The model under review builds one solid part; all positions refer to its coordinate system, in mm. A direction names the side the tool comes from. Coordinates: 2 decimals unless noted, no trailing zeros. Write each loop counter-clockwise with the first axis right and the second up, starting at its lowest first coordinate (ties: lowest second). Pieces come first, ordered by that corner, then holes.
1) Add section D-D, the plane y = 3.5. State the section outline as (x, z) points.
2) Machinability: for faces 5 (the flat face through (53, 4, 4.25)), 6 (the flat face through (53, 14.662, 3)), 7 (the flat face through (-9.287, 4, 1)), which of the approach directions +Z, -Z, +X, -X, +Y, -Y give a long, thin tool a straight path to every point of the face, cutting with its end or side? Answer none if there is none.
3) Mouldability with a two-part tool opening along Y and no side actions: class faces 1 (the flat face through (-3, 24.162, 6)), 2 (the cylindrical face through (-5.966, 30.025, 0.863)), 3 (the flat face through (24, 5, 0)), 4 (the cylindrical face through (52.034, 30.025, 0.863)) as released by +Y, released by -Y, zero draft, split by the parting line, or undercut.
4) For P1, Ø3, axis at x = 53.5, z = 3.5, coming from the -Y side; P2, Ø1, axis at x = 14.5, y = 16.5, coming from the -Z side; P3, Ø2.5, axis at x = -5.5, z = 7, coming from the -Y side; P4, Ø2, axis at x = 8.5, y = -7, coming from the +Z side, all flat-tipped, find the tip position at first contact; note any pin that passes through.
5) For line 1 (Z direction, x = 4, y = 11); line 2 (X direction, y = 15, z = 4.75); line 3 (X direction, y = -5, z = 1.5), list the stretches that pass through material, from the lowest coordinate up.
6) Add section A-A, the plane y = 20.5. State the section outline as (x, z) points.
7) Add section C-C, the plane x = 7. State the section outline as (y, z) points, then the cut area to 3 significant figures.
8) Add section B-B, the plane z = 2.5. State the section outline as (x, y) points.
from build123d import *

# Parameters (mm, degrees)
SKETCH003_W  = 5.5
SKETCH003_H  = 20.7
PAD002_DEPTH = 2.5
SKETCH_W     = 14
SKETCH_H     = 13.5
PAD001_DEPTH = 9
SKETCH002_R  = 1.375
PAD_DEPTH    = 1.75


with BuildPart() as displayport:
    # Sketch003 (on Face1 of ShapeBinder001) → Pad002 (new body)
    with BuildSketch(Plane.XY.offset(1.75)):
        with Locations((52.9627, 4.312003)):
            Rectangle(SKETCH003_W, SKETCH003_H)
    extrude(amount=PAD002_DEPTH)


with BuildPart() as usb:
    # Sketch (on Face1 of ShapeBinder) → Pad001 (new body)
    with BuildSketch(Plane.XY.offset(1.75)):
        with Locations((-3.2873, 17.412003)):
            Rectangle(SKETCH_W, SKETCH_H)
    extrude(amount=PAD001_DEPTH)


with BuildPart() as fusion001:
    # Sketch002 → Pad (new body)
    with BuildSketch(Plane.XY):
        with BuildLine():
            Line((-6.2873, 32.162003), (52.7127, 32.162003))
            ThreePointArc((55.7127, 29.162003), (54.83402, 31.283323), (52.7127, 32.162003))
            Line((55.7127, 29.162003), (55.7127, -20.837997))
            ThreePointArc((52.7127, -23.837997), (54.83402, -22.959317), (55.7127, -20.837997))
            Line((52.7127, -23.837997), (-6.2873, -23.837997))
            ThreePointArc((-9.2873, -20.837997), (-8.40862, -22.959317), (-6.2873, -23.837997))
            Line((-9.2873, -20.837997), (-9.2873, 29.162003))
            ThreePointArc((-6.2873, 32.162003), (-8.40862, 31.283323), (-9.2873, 29.162003))
        make_face()
        with Locations((-5.7873, 28.662003)):
            Circle(SKETCH002_R, mode=Mode.SUBTRACT)
        with Locations((-5.7873, -20.337997)):
            Circle(SKETCH002_R, mode=Mode.SUBTRACT)
        with Locations((52.2127, -20.337997)):
            Circle(SKETCH002_R, mode=Mode.SUBTRACT)
        with Locations((52.2127, 28.662003)):
            Circle(SKETCH002_R, mode=Mode.SUBTRACT)
    extrude(amount=PAD_DEPTH)

    # Fusion: union usb
    add(usb.part)

    # Fusion001: union displayport
    add(displayport.part)


solid = fusion001.part
Geometry results:
1. outline: (-9.29, 0) - (55.71, 0) - (55.71, 4.25) - (50.21, 4.25) - (50.21, 1.75) - (-9.29, 1.75) - close
2. face 5: +Z, +X, +Y, -Y
2. face 6: +Z, +X, +Y
2. face 7: -Z, -X, +Y, -Y
3. face 1: released by +Y
3. face 2: undercut
3. face 3: zero draft
3. face 4: undercut
4. P1: stops at y = -6.04
4. P2: stops at z = 0
4. P3: stops at y = 10.66
4. P4: stops at z = 1.75
5. line 1: z = 0 to 1.75
5. line 2: x = -10.29 to 3.71
5. line 3: x = -9.29 to 55.71
6. outline: (-10.29, 1.75) - (-9.29, 1.75) - (-9.29, 0) - (55.71, 0) - (55.71, 1.75) - (3.71, 1.75) - (3.71, 10.75) - (-10.29, 10.75) - close
7. outline: (-23.84, 0) - (32.16, 0) - (32.16, 1.75) - (-23.84, 1.75) - close
7. area: 98.0 mm2
8. outline: (-10.29, 10.66) - (3.71, 10.66) - (3.71, 24.16) - (-10.29, 24.16) - close; (50.21, -6.04) - (55.71, -6.04) - (55.71, 14.66) - (50.21, 14.66) - close
